from build123d import *

# Parameters (mm, degrees)
F2_W     = 0.225
F2_H     = 0.6141559725
F3_DEPTH = 12.5
F4_R     = 0.075


with BuildPart() as f1:
    # F0 (on Top) → F1 (revolve)
    with BuildSketch(Plane.XY):
        with BuildLine():
            Line((-101.5040925145, -14.4654285704), (-101.5040925145, -9.9654285704))
            ThreePointArc((-101.5040925145, -9.9654285704), (-103.0950827722, -10.6244383127), (-103.7540925145, -12.2154285704))
            ThreePointArc((-103.7540925145, -12.2154285704), (-103.0950827722, -13.8064188281), (-101.5040925145, -14.4654285704))
        make_face()
        with BuildLine():
            Line((-101.5040925145, -17.8512725979), (-101.5040925145, -14.4654285704))
            ThreePointArc((-101.5040925145, -14.4654285704), (-103.0950827722, -13.8064188281), (-103.7540925145, -12.2154285704))
            Line((-103.7540925145, -12.2154285704), (-103.7540925145, -17.8512725979))
            Line((-103.7540925145, -17.8512725979), (-101.5040925145, -17.8512725979))
        make_face()
        Polygon((-101.5040925145, -18.4654285704), (-101.5040925145, -17.8512725979), (-103.7540925145, -17.8512725979), (-104.0040925145, -17.8512725979), (-104.0040925145, -18.4654285704), align=None)
    revolve(axis=Axis((-101.5040925145, -14.2154285704, 0), (0, -1, 0)))

    # F2 (on Top) → F3 (cut, symmetric)
    with BuildSketch(Plane.XY):
        with Locations((-99.1165925145, -18.1583505842)):
            Rectangle(F2_W, F2_H)
    extrude(amount=F3_DEPTH, both=True, mode=Mode.SUBTRACT)

    # F4
    f4_edges = [f1.edges().sort_by_distance(p)[0] for p in [
        (-104.004093, -17.851273, 0),
        (-99.229093, -17.851273, 0),
        (-99.229093, -18.158351, 1.036521),
        (-99.229093, -18.158351, -1.036521),
    ]]
    fillet(f4_edges, radius=F4_R)


solid = f1.part
Read the model definition and answer for the solid it produces. Units are mm, in the model's axes. A direction names the side the tool comes from. Round coordinates to 2 decimals unless told otherwise and drop trailing zeros. Write each loop counter-clockwise with the first axis right and the second up, starting at its lowest first coordinate (ties: lowest second). Pieces come first, ordered by that corner, then holes. Notation, with made-up numbers: (-11.75, 36) - (-3.75, 36) arc R21 ccw to (-3.75, 40) - close; hole circle Ø3 at (33, -17.75). An arc over 180 degrees is marked (long way). One line per question, with ' | ' between items. Start each with the question number.
1. Find the intervals of material crossed by probe 1 along Y at (x, z) = (-100.6, -2.15); probe 2 along X at (y, z) = (-11, -1.5); probe 3 along X at (y, z) = (-14, 1.3), in increasing order. Write a range as [from, to].
2. Section A-A (y = -17.5) is taken. Determine the outline of the cut face in (x, z), and give its area (3 significant figures).
3. Each of these flat-tipped pins is pushed along its axis until it touches: pin 1 (3 mm diameter, centred on y = -16, z = 1, fed in from -X); pin 2 (1 mm diameter, centred on y = -11, z = -2, fed in from +X); pin 3 (1.5 mm diameter, centred on x = -101.5, y = -13, fed in from -Z). Where does it stop, or does it pass through?
4. For faces 1 (the face through (-104.002, -18.2, 0.095)), 2 (the face through (-103.583, -15.073, 0.862)), determine the directions among +Z, -Z, +X, -X, +Y, -Y from which every point of the face is accessible in a straight line to the end or side of a thin tool.
Filled in:
1) probe 1: [-18.47, -17.85] | probe 2: [-102.66, -100.35] | probe 3: [-103.34, -99.67]
2) outline: circle Ø4.5 at (-101.5, 0) | area: 15.9 mm²
3) pin 1: x = -103.75 | pin 2: x = -100.21 | pin 3: z = -2.25
4) face 1: +Y, -Y | face 2: +Y
